```python
from build123d import *

# Parameters (mm, degrees)
SKETCH1_R           = 4.7625
BOSS_EXTRUDE1_DEPTH = 50.8
BOSS_EXTRUDE2_DEPTH = 5


with BuildPart() as part:
    # Sketch1 → Boss-Extrude1 (new body)
    with BuildSketch(Plane(origin=(0, 0, 0), x_dir=(0, 0, -1), z_dir=(1, 0, 0))):
        Circle(SKETCH1_R)
    extrude(amount=BOSS_EXTRUDE1_DEPTH)

    # Sketch2 → Boss-Extrude2 (add)
    with BuildSketch(Plane.ZY):
        Polygon((8.082903769, 0), (4.041451884, 7), (-4.041451884, 7), (-8.082903769, 0), (-4.041451884, -7), (4.041451884, -7), align=None)
    extrude(amount=BOSS_EXTRUDE2_DEPTH)


solid = part.part
```
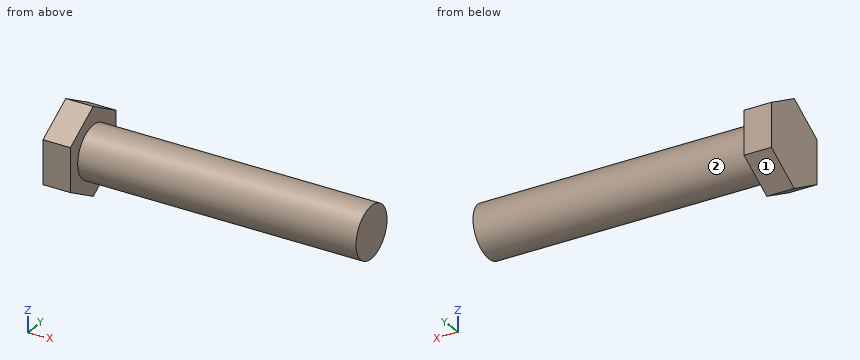
Model file for the job. Use its own axes, mm. Face numbers are marked on the shaded views. A direction names the side the tool comes from. Coordinates: 2 decimals unless noted, no trailing zeros. Loops run counter-clockwise (first coordinate to the right, second up) from the corner with the lowest first, then second, coordinate; pieces in that order, holes last. Notation, with made-up numbers: (-16.5, 2) - (40.5, 2) arc R22 ccw to (40.5, 21) - close; hole circle Ø6 at (27.5, 77). An arc over 180 degrees is marked (long way). Answer as a JSON object with one key per item and string values. Group by question number.
(1) Cut at D-D (y = -5.5). Give the cut face in (x, z), then the cut area to 3 significant figures.
(2) Cut at A-A (z = 0). Give the cut face in (x, y), then the cut area to 3 significant figures.
(3) Tool access for the marked faces 1 and 2: list every direction of +Z, -Z, +X, -X, +Y, -Y with a clear straight run to the whole face (end or side of a thin tool).
(4) Cut at C-C (y = 2.75). Give the cut face in (x, z).
(5) Flat gauge pins, fed straight in: pin 1 (2 mm diameter, centred on x = 22, z = 2, fed in from +Y); pin 2 (6 mm diameter, centred on x = 35, z = 0, fed in from -Y); pin 3 (6 mm diameter, centred on x = 17.5, z = -1.5, fed in from +Y). Where does each tip first touch, or does it go through?
(6) Probe line 1 along X through (y, z) = (6, -2.5); line 2 along Z through (x, y) = (9, -0.25); line 3 along Y through (x, z) = (21, 2.5). List the from-to ranges inside material, lowest first.
(7) Cut at B-B (x = 18). Give the cut face in (y, z) (1 decimal).
Geometry says:
{
 "1": {"outline": "(-5, -4.91) - (0, -4.91) - (0, 4.91) - (-5, 4.91) - close", "area": "49.1 mm^2"},
 "2": {"outline": "(-5, -7) - (0, -7) - (0, -4.76) - (50.8, -4.76) - (50.8, 4.76) - (0, 4.76) - (0, 7) - (-5, 7) - close", "area": "554 mm^2"},
 "3": {"face 1": "-Z, +X, -X, +Y", "face 2": "+X"},
 "4": {"outline": "(-5, -6.5) - (0, -6.5) - (0, -3.89) - (50.8, -3.89) - (50.8, 3.89) - (0, 3.89) - (0, 6.5) - (-5, 6.5) - close"},
 "5": {"pin 1": "stops at y = 4.66", "pin 2": "stops at y = -4.76", "pin 3": "stops at y = 4.76"},
 "6": {"line 1": "x = -5 to 0", "line 2": "z = -4.76 to 4.76", "line 3": "y = -4.05 to 4.05"},
 "7": {"outline": "circle Ø9.5 at (0, 0)"}
}
